Verification items for the finished model (mm, model axes). Face numbers are marked on the shaded views. A direction names the side the tool comes from. Round coordinates to 2 decimals unless told otherwise and drop trailing zeros. Loops run counter-clockwise (first coordinate to the right, second up) from the corner with the lowest first, then second, coordinate; pieces in that order, holes last. Notation, with made-up numbers: (-10.75, 15.5) -> (43.25, 15.5) arc R28 cw to (43.25, 45.5) -> close; hole circle Ø10 at (52.25, 23). An arc over 180 degrees is marked (long way). Use CSV: the item, a comma, the result in double quotes. Start each with the question number.
Autodesk Fusion 360 part; units mm, degrees
sketch "Szkic1" plane through (0, 0, 0) normal (0, 0, 1) x (1, 0, 0)
  line L0 (-23.5, -30) -> (30, -30)
  line L1 (-23.5, 0) -> (-23.5, -30)
  line L2 (30, -30) -> (30, 0)
  line L3 (30, 0) -> (-23.5, 0)
  line L4 (5, -5) -> (7, -5)
  line L5 (18.5, -5) -> (18.5, -30)
  line L6 (18.5, -5) -> (18.5, 0)
  circle A0 centre (5, -25) radius 1.75
  circle A1 centre (5, -5) radius 1.75
  circle A2 centre (-10, -25) radius 1.75
  circle A3 centre (-10, -5) radius 1.75
  circle A4 centre (-10, -25) radius 3.5
  circle A5 centre (5, -25) radius 3.5
  circle A6 centre (5, -5) radius 3.5
  circle A7 centre (-10, -5) radius 3.5
  line L7 (-10, -5) -> (-9, -5)
  line L8 (-9, -5) -> (-2, -5)
  line L9 (-14, -10) -> (-14, -19)
  line L10 (10, -21) -> (10, -9)
  line L11 (10, -9) -> (-14, -9)
  line L12 (-14, -9) -> (-14, -10)
  line L13 (-14, -19) -> (-14, -21)
  line L14 (-14, -21) -> (10, -21)
  dimension "d1" = 13.5
  dimension "d3" = 3.5
  dimension "d4" = 3.5
  dimension "d5" = 3.5
  dimension "d6" = 3.5
  dimension "d7" = 7
  dimension "d8" = 7
  dimension "d9" = 7
  dimension "d10" = 7
extrude "Wyciągnięcie proste1" add sketch "Szkic1" along normal blind 7 contours L0 L1 L3 L5 L6
extrude "Wyciągnięcie proste2" add sketch "Szkic1" along normal blind 20 contours L9 L10 L11 L12 L13 L14
extrude "Wyciągnięcie proste3" add sketch "Szkic1" along normal blind 4 contours A7 | A4 | A5 | A6
extrude "Wyciągnięcie proste4" add 1 faces at (-6, -13, 20) along direction (0, 0, 1) blind 5
sketch "Szkic2" plane through (10, 0, 0) normal (1, 0, 0) x (0, 1, 0)
  line L0 (-21, 7) -> (-9, 7)
  line L1 (-9, 7) -> (-9, 25)
  line L2 (-9, 25) -> (-21, 25)
  line L3 (-21, 25) -> (-21, 7)
  circle A0 centre (-15, 20) radius 3.25
  dimension "d19" = 6.5
extrude "Wyciągnięcie proste5" add sketch "Szkic2" along normal blind 3 contours L0 L1 L2 L3 | A0
extrude "Wyciągnięcie proste6" add 1 faces at (-14, -17, 19) along direction (-1, 0, 0) blind 3
extrude "Wyciągnięcie proste7" cut sketch "Szkic2" against normal blind 24 contours L0 L1 L2 L3 | A0
extrude "Wyciągnięcie proste8" add sketch "Szkic2" against normal blind 22 contours A0
extrude "Wyciągnięcie proste9" add 1 faces at (-12, -14.06, 19.6878) along direction (-1, 0, 0) blind 3
extrude "Wyciągnięcie proste10" cut sketch "Szkic2" against normal blind 21.5 contours A0
extrude "Wyciągnięcie proste11" add sketch "Szkic2" against normal blind 2.5 contours A0
extrude "Wyciągnięcie proste12" cut 1 faces at (-14, -14.919, 10.253) along direction (-1, 0, 0) blind 2
extrude "Wyciągnięcie proste13" cut 1 faces at (10, -14.919, 10.253) along direction (1, 0, 0) blind 2
extrude "Wyciągnięcie proste14" cut 1 faces at (7.5, -14.06, 19.6878) along direction (1, 0, 0) blind 2
extrude "Wyciągnięcie proste15" cut 1 faces at (-11.5, -14.06, 19.6878) along direction (-1, 0, 0) blind 2
extrude "Wyciągnięcie proste16" add 1 faces at (-17, -17, 19) along direction (-1, 0, 0) blind 2
extrude "Wyciągnięcie proste17" add 1 faces at (13, -13, 13) along direction (1, 0, 0) blind 3
extrude "Wyciągnięcie proste18" add 1 faces at (-19, -17, 19) along direction (-1, 0, 0) blind 1
chamfer "Fazowanie1" distance 3 angle 45 1 edges at (-20, -15, 7)
chamfer "Fazowanie2" distance 2 angle 45 1 edges at (16, -15, 7)
sketch "Szkic3" plane through (9.5, 0, 0) normal (-1, 0, 0) x (0, -1, 0)
  circle A0 centre (15, 20) radius 3.25
  circle A1 centre (15, 20) radius 2.75
  dimension "d50" = 5.5
extrude "Wyciągnięcie proste19" cut sketch "Szkic3" against normal blind 2.5
extrude "Wyciągnięcie proste20" cut sketch "Szkic3" along normal blind 25.5
equation "d26 = 2 mm - 24 mm"
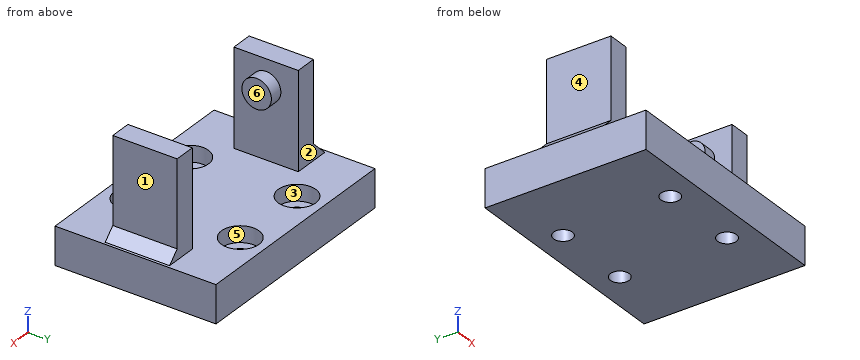
Q1. Tool access check on the marked faces 4, 5 and 6. Record the directions out of +Z, -Z, +X, -X, +Y, -Y that give a thin tool (end or side, any length) a straight path to the whole face; none if there is none.
Q2. Cross-section at C-C (z = 8.5). Record the boundary of the cut face in (x, y).
Q3. Cross-section at B-B (y = -25). Record the boundary of the cut face in (x, z).
Q4. Cross-section at D-D (x = 11). Record the boundary of the cut face in (y, z).
Q5. Depth check by flat-ended pin: pin 1 Ø5 at (x, y) = (-9, -24) entering from +Z; pin 2 Ø3 at (y, z) = (-16, 19) entering from +X; pin 3 Ø3.5 at (x, y) = (-9.5, -3.5) entering from +Z; pin 4 Ø3 at (x, y) = (5, -5) entering from -Z. Enter the tip coordinate at first touch or a pass-through.
Q6. Thickness scan on L1, parallel to Y at x = -10, z = 3; L2, parallel to Y at x = 5, z = 4.85; L3, parallel to X at y = -15.25, z = 16. Record the ranges inside material, lowest first. Write a range as from..to.
Q7. Release check for a two-part mould opening along X. For the marked faces 1, 2 and 3 record: +X half, -X half, draft (parallel to the pull), parting line (faces both ways), or undercut.
Q8. Cross-section at A-A (x = 5). Record the boundary of the cut face in (y, z), and give its area (3 significant figures).
Answer list:
1,face 4,"+Z, -X, +Y, -Y"
1,face 5,"+Z"
1,face 6,"+Z, +Y, -Y"
2,outline,"(-21.5, -21) -> (-16, -21) -> (-16, -9) -> (-21.5, -9) -> close; (12, -21) -> (16.5, -21) -> (16.5, -9) -> (12, -9) -> close"
3,outline,"(-23.5, 0) -> (-11.75, 0) -> (-11.75, 4) -> (-13.5, 4) -> (-13.5, 7) -> (-23.5, 7) -> close; (-8.25, 0) -> (3.25, 0) -> (3.25, 4) -> (1.5, 4) -> (1.5, 7) -> (-6.5, 7) -> (-6.5, 4) -> (-8.25, 4) -> close; (6.75, 0) -> (18.5, 0) -> (18.5, 7) -> (8.5, 7) -> (8.5, 4) -> (6.75, 4) -> close"
4,outline,"(-30, 0) -> (0, 0) -> (0, 7) -> (-30, 7) -> close; circle Ø5.5 at (-15, 20)"
5,pin 1,"stops at z = 7"
5,pin 2,"stops at x = 16"
5,pin 3,"stops at z = 4"
5,pin 4,"passes through"
6,L1,"y = -30..-26.75, -23.25..-6.75, -3.25..0"
6,L2,"y = -30..-28.5, -21.5..-8.5, -1.5..0"
6,L3,"x = -20..-16, 12..16"
7,face 1,"+X half"
7,face 2,"draft"
7,face 3,"undercut"
8,outline,"(-30, 0) -> (-26.75, 0) -> (-26.75, 4) -> (-28.5, 4) -> (-28.5, 7) -> (-30, 7) -> close; (-23.25, 0) -> (-6.75, 0) -> (-6.75, 4) -> (-8.5, 4) -> (-8.5, 7) -> (-21.5, 7) -> (-21.5, 4) -> (-23.25, 4) -> close; (-3.25, 0) -> (0, 0) -> (0, 7) -> (-1.5, 7) -> (-1.5, 4) -> (-3.25, 4) -> close"
8,area,"140 mm2"
